Study the drawing (mm; zero at the part's minimum x, y, z) and answer. A direction names the side the tool comes from. Coordinates: 2 decimals unless noted, no trailing zeros. Write each loop counter-clockwise with the first axis right and the second up, starting at its lowest first coordinate (ties: lowest second). Pieces come first, ordered by that corner, then holes. Notation, with made-up numbers: M -29,-8.75 L -4,-8.75 A29 cw -4,19.25 Z; hole C 30,63.25 d6. An arc over 180 degrees is marked long. Answer as CSV lines item,"result". Start each with the question number.
(1) A cutting plane is placed at D-D on x = 92. Give the vertices of the cut face in (y, z), then the cut area to 3 significant figures.
(2) A cutting plane is placed at C-C on y = 77.5. Give the vertices of the cut face in (x, z), then the cut area to 3 significant figures.
(3) Find the intervals of material crossed by L1, parallel to X at y = 63.5, z = 84; L2, parallel to Y at x = 5.5, z = 78.5; L3, parallel to Y at x = 81, z = 100, in increasing order. Write a range as [from, to].
(4) A cutting plane is placed at A-A on y = 22.5. Give the vertices of the cut face in (x, z).
(5) For the marked faces 5 and 6, determine the directions among +Z, -Z, +X, -X, +Y, -Y from which every point of the face is accessible in a straight line to the end or side of a thin tool.
(6) A cutting plane is placed at B-B on z = 60. Give the vertices of the cut face in (x, y).
(7) Flat-ended cylindrical pins translate along their axes: P1, Ø10, axis at x = 77.5, z = 29.5, coming from the +Y side; P2, Ø3, axis at x = 36, y = 43.5, coming from the -Z side; P3, Ø1, axis at x = 13, z = 40.5, coming from the -Y side; P4, Ø11, axis at x = 86, y = 36.5, coming from the +Z side. Find the tip coordinate at first contact, or state that the pin passes through.
(8) The mould has two halves that part along X. Classify the marked faces 1, 2, 3 and 4: released by +X, released by -X, zero draft, split by the parting line, or undercut.
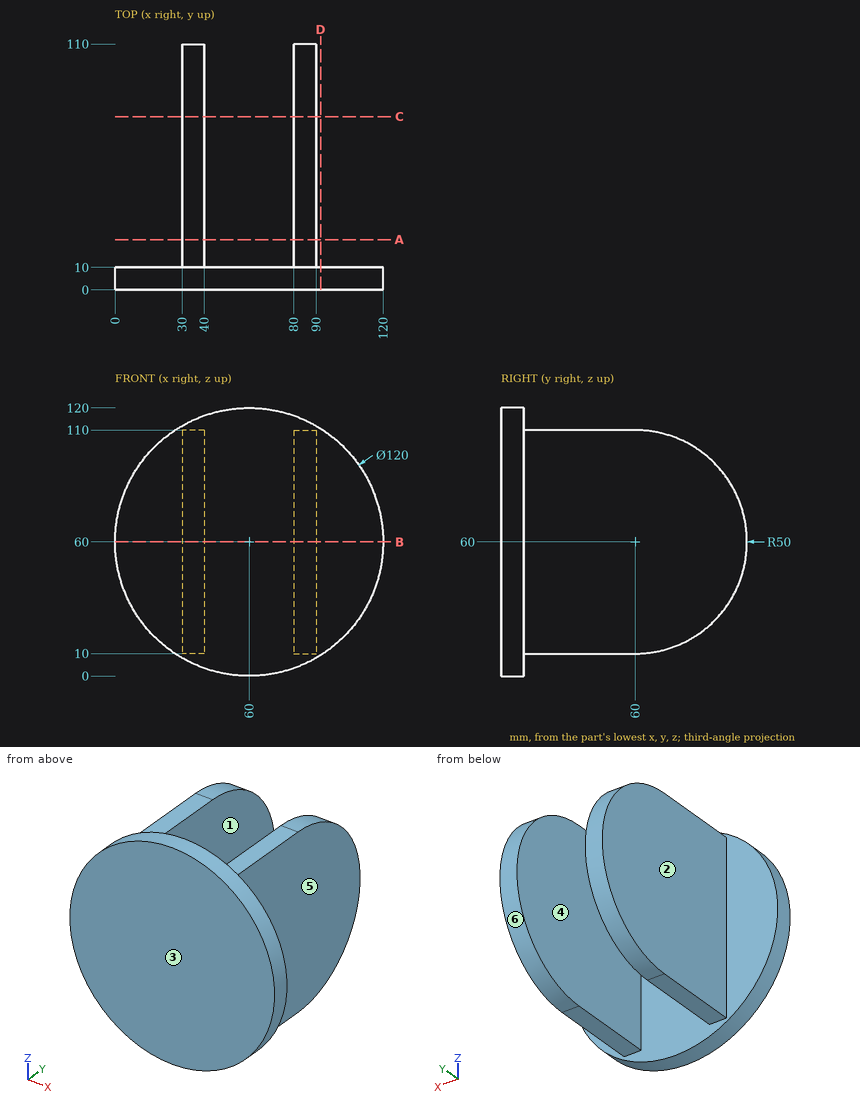
Here are the results:
1,outline,"M 0,9.25 L 10,9.25 L 10,110.75 L 0,110.75 Z"
1,area,"1,020 mm^2"
2,outline,"M 30,13.16 L 40,13.16 L 40,106.84 L 30,106.84 Z; M 80,13.16 L 90,13.16 L 90,106.84 L 80,106.84 Z"
2,area,"1,870 mm^2"
3,L1,"x = [30, 40], [80, 90]"
3,L2,"y = [0, 10]"
3,L3,"y = [0, 90]"
4,outline,"M 30,10 L 40,10 L 40,110 L 30,110 Z; M 80,10 L 90,10 L 90,110 L 80,110 Z"
5,face 5,"+Z, -Z, +X, +Y"
5,face 6,"+X, -X, +Y"
6,outline,"M 0,0 L 120,0 L 120,10 L 90,10 L 90,110 L 80,110 L 80,10 L 40,10 L 40,110 L 30,110 L 30,10 L 0,10 Z"
7,P1,"stops at y = 102.6"
7,P2,"stops at z = 10"
7,P3,"stops at y = 0"
7,P4,"stops at z = 110"
8,face 1,"undercut"
8,face 2,"released by -X"
8,face 3,"zero draft"
8,face 4,"undercut"
